Check sheet for the modelled part. Datum: model origin and axes. Units: mm. Face numbers are marked on the shaded views. A direction names the side the tool comes from. Give positions to 0.01 mm unless a question says otherwise; leave off trailing zeros. Order: outer loops, then holes, each group sorted by start corner. A loop starts at its lowest first (then second) coordinate and runs counter-clockwise, first axis right, second up.
Item 1: Sectioned sample at A-A on z = -61. Record the boundary of the cut face in (x, y), and give its area (3 significant figures).
Item 2: Sectioned sample at B-B on x = 316. Record the boundary of the cut face in (y, z), and give its area (3 significant figures).
Item 3: Gauge pin test, flat ends, axial feed: P1, Ø2, axis at x = -116.5, z = -30, coming from the -Y side; P2, Ø12, axis at y = -252, z = -27.5, coming from the -X side; P3, Ø4, axis at y = 80, z = -61, coming from the +X side. Record the tip position at first contact, or that the pin passes through.
Item 4: Release check for a two-part mould opening along Y. For the marked faces 3, 4, 5 and 6 record: released by +Y, released by -Y, zero draft, split by the parting line, or undercut.
Item 5: Material ranges on line 1 along Z through (x, y) = (67.5, -322); line 2 along Y through (x, z) = (102.5, -41.5); line 3 along X through (y, z) = (-144, -18), recorded low to high.
Item 6: Sectioned sample at C-C on y = -275. Record the boundary of the cut face in (x, z), and give its area (3 significant figures).
Item 7: Access from +Z, -Z, +X, -X, +Y, -Y to the whole of each face (thin tool, end or side, straight path). Record for the marked faces 1 and 2.
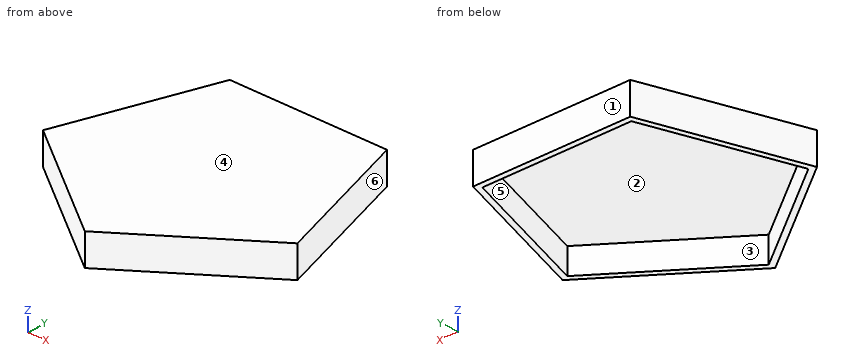
from build123d import *

# Parameters (mm, degrees)
F1_DEPTH = 18
F3_DEPTH = 80


with BuildPart() as f1:
    # F0 (on Top) → F1 (new body)
    with BuildSketch(Plane.XY):
        Polygon((444.386186, -117.506794), (289.877689, 358.021464), (-210.122311, 358.021464), (-364.630808, -117.506794), (39.877689, -411.39942), align=None)
    extrude(amount=F1_DEPTH)

    # F2 (on face) → F3 (join)
    with BuildSketch(Plane(origin=(0, 0, 0), x_dir=(1, 0, 0), z_dir=(0, 0, -1))):
        Polygon((-364.630808, 117.506794), (-210.122311, -358.021464), (289.877689, -358.021464), (444.386186, 117.506794), (39.877689, 411.39942), align=None)
        Polygon((276.799923, -340.021464), (-197.044546, -340.021464), (-343.470539, 110.631406), (39.877689, 389.150196), (423.225917, 110.631406), align=None, mode=Mode.SUBTRACT)
    extrude(amount=F3_DEPTH)


solid = f1.part
Report:
1. outline: (-364.63, -117.51) - (39.88, -411.4) - (444.39, -117.51) - (289.88, 358.02) - (-210.12, 358.02) - close; hole (-343.47, -110.63) - (39.88, -389.15) - (423.23, -110.63) - (276.8, 340.02) - (-197.04, 340.02) - close
1. area: 43,800 mm2
2. outline: (-210.78, -80) - (-188.54, -80) - (-188.54, 0) - (219.38, 0) - (219.38, -80) - (277.63, -80) - (277.63, 18) - (-210.78, 18) - close
2. area: 15,200 mm2
3. P1: stops at y = -298.51
3. P2: stops at x = -187.78
3. P3: stops at x = 380.86
4. face 3: undercut
4. face 4: zero draft
4. face 5: undercut
4. face 6: released by +Y
5. line 1: z = 0 to 18
5. line 2: y = -365.9 to -343.65, 340.02 to 358.02
5. line 3: x = -328.17 to -297.54, 377.3 to 407.92
6. outline: (-147.86, -80) - (-117.24, -80) - (-117.24, 0) - (196.99, 0) - (196.99, -80) - (227.62, -80) - (227.62, 18) - (-147.86, 18) - close
6. area: 11,700 mm2
7. face 1: +Z, -Z, +X, -X, +Y
7. face 2: -Z
